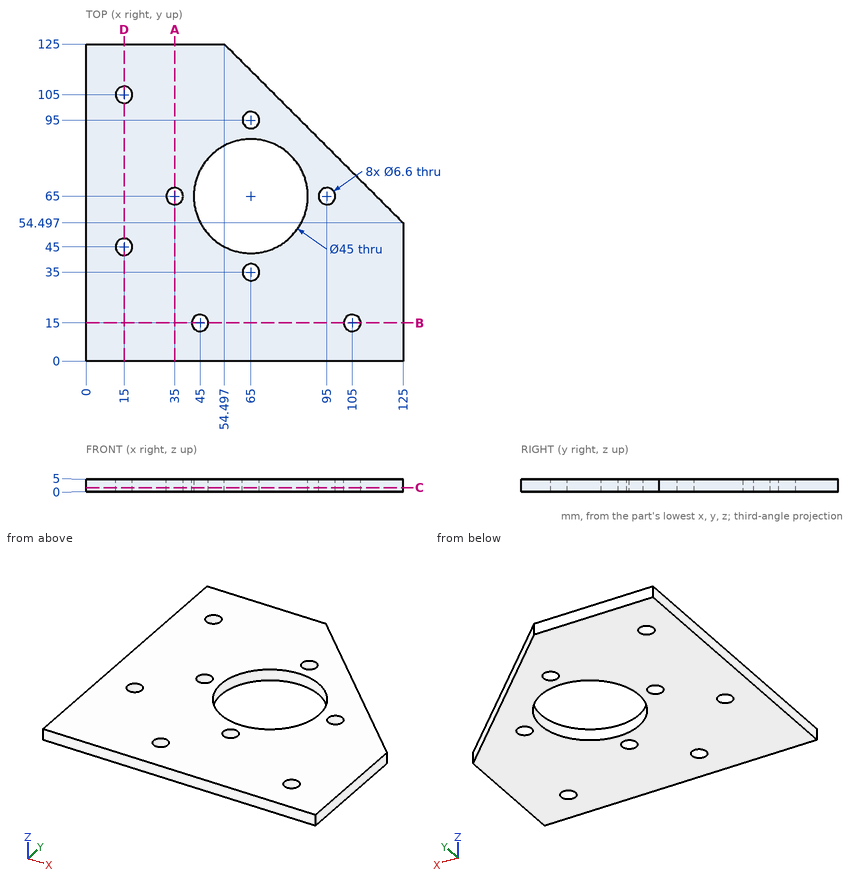
Study the drawing (mm; zero at the part's minimum x, y, z) and answer. Give positions to 0.01 mm unless a question says otherwise; leave off trailing zeros. Loops run counter-clockwise (first coordinate to the right, second up) from the corner with the lowest first, then second, coordinate; pieces in that order, holes last. Notation, with made-up numbers: M -20.5,4 L 10.5,4 A35 cw 10.5,40 Z; hole C 53,76.25 d11. An arc over 180 degrees is marked long. One line per item, written item: value.
1. Each of these flat-tipped pins is pushed along its axis until it touches: P1, Ø3, axis at y = 82, z = 3.5, coming from the +X side; P2, Ø10.5, axis at x = 15, y = 105, coming from the -Z side; P3, Ø5.5, axis at x = 95, y = 65, coming from the -Z side. Where does it stop, or does it pass through?
Found:
P1: x = 99
P2: z = 0
P3: through
2. Section A-A on x = 35 is taken. Determine the outline of the cut face in (y, z), plus the area to 3 significant figures.
Found:
outline: M 0,0 L 61.7,0 L 61.7,5 L 0,5 Z; M 68.3,0 L 125,0 L 125,5 L 68.3,5 Z
area: 592 mm^2
3. Find the intervals of material crossed by probe 1 along Y at (x, z) = (15, 2.4); probe 2 along Y at (x, z) = (65, 2.15) (1 decimal); probe 3 along X at (y, z) = (67.5, 0.95) (1 decimal), in increasing order.
Found:
probe 1: 0 to 41.7, 48.3 to 101.7, 108.3 to 125
probe 2: 0 to 31.7, 38.3 to 42.5, 87.5 to 91.7, 98.3 to 114.5
probe 3: 0 to 32.8, 37.2 to 42.6, 87.4 to 92.8, 97.2 to 112
4. Section C-C on z = 1.6 is taken. State how many separate pieces and enclosed holes the cut face has, plus the area to 3 significant figures.
Found:
separate pieces: 1
enclosed holes: 9
area: 11,300 mm^2
5. Section B-B on y = 15 is taken. Determine the outline of the cut face in (x, z).
Found:
outline: M 0,0 L 41.7,0 L 41.7,5 L 0,5 Z; M 48.3,0 L 101.7,0 L 101.7,5 L 48.3,5 Z; M 108.3,0 L 125,0 L 125,5 L 108.3,5 Z
